Source: CAD feature listing. Evaluate the final solid. Frame: model axes, mm. A direction names the side the tool comes from. Round coordinates to 2 decimals unless told otherwise and drop trailing zeros. Write each loop counter-clockwise with the first axis right and the second up, starting at its lowest first coordinate (ties: lowest second). Pieces come first, ordered by that corner, then holes. Notation, with made-up numbers: M 62.5,70.25 L 100.5,70.25 A14 ccw 100.5,84.25 Z; hole C -18.5,5.25 d4. An arc over 180 degrees is marked long. Answer in a Markdown table with one row per item.
from build123d import *

# Parameters (mm, degrees)
BOX005_W                  = 41
BOX005_H                  = 42
BOX005_DEPTH              = 40
BOX004_W                  = 7
BOX004_H                  = 17
BOX004_DEPTH              = 10
CYLINDER003_R             = 2.5
CYLINDER003_DEPTH         = 25
CYLINDER002_R             = 2.5
CYLINDER002_DEPTH         = 4
BOX006_W                  = 45
BOX006_H                  = 3
BOX006_DEPTH              = 8
BOX007_W                  = 3
BOX007_H                  = 50
BOX007_DEPTH              = 8
BOX003_W                  = 45
BOX003_H                  = 50
BOX003_DEPTH              = 3
FUSION002_ROLL_ANGLE      = 90
FUSION002_PLACEMENT_ANGLE = 90


with BuildPart() as base_motor:
    # Box005 → Box005 (new body)
    with BuildSketch(Plane(origin=(4, 4, 0), x_dir=(1, 0, 0), z_dir=(0, 0, 1))):
        with Locations((20.5, 21)):
            Rectangle(BOX005_W, BOX005_H)
    extrude(amount=BOX005_DEPTH)


with BuildPart() as obj1:
    # Box004 → Box004 (new body)
    with BuildSketch(Plane(origin=(45, 16.5, 0), x_dir=(1, 0, 0), z_dir=(0, 0, 1))):
        with Locations((3.5, 8.5)):
            Rectangle(BOX004_W, BOX004_H)
    extrude(amount=BOX004_DEPTH)


with BuildPart() as motor:
    # Cylinder003 → Cylinder003 (new body)
    with BuildSketch(Plane(origin=(25, 25, 43), x_dir=(1, 0, 0), z_dir=(0, 0, 1))):
        Circle(CYLINDER003_R)
    extrude(amount=CYLINDER003_DEPTH)

    # Fusion003: union base motor, obj1
    add(base_motor.part)
    add(obj1.part)


with BuildPart() as obj2:
    # Cylinder002 → Cylinder002 (new body)
    with BuildSketch(Plane(origin=(10, 10, 43), x_dir=(1, 0, 0), z_dir=(0, 0, 1))):
        Circle(CYLINDER002_R)
    extrude(amount=CYLINDER002_DEPTH)


with BuildPart() as obj3:
    # Link003 base: copy of obj2
    add(obj2.part)


with BuildPart() as obj3_1:
    # Link003 placement: moved
    add(obj3.part.moved(Location((30, 30, 0))))


with BuildPart() as obj4:
    # Link004 base: copy of obj2
    add(obj2.part)


with BuildPart() as obj4_1:
    # Link004 placement: moved
    add(obj4.part.moved(Location((30, 0, 0))))


with BuildPart() as obj5:
    # Link005 base: copy of obj2
    add(obj2.part)


with BuildPart() as obj5_1:
    # Link005 placement: moved
    add(obj5.part.moved(Location((0, 30, 0))))


with BuildPart() as obj6:
    # Box006 → Box006 (new body)
    with BuildSketch(Plane.XY.offset(32)):
        with Locations((22.5, 1.5)):
            Rectangle(BOX006_W, BOX006_H)
    extrude(amount=BOX006_DEPTH)


with BuildPart() as lateral_der:
    # Link006 base: copy of obj6
    add(obj6.part)


with BuildPart() as lateral_der_1:
    # Link006 placement: moved
    add(lateral_der.part.moved(Location((0, 47, 0))))


with BuildPart() as obj7:
    # Box007 → Box007 (new body)
    with BuildSketch(Plane.XY.offset(32)):
        with Locations((1.5, 25)):
            Rectangle(BOX007_W, BOX007_H)
    extrude(amount=BOX007_DEPTH)


with BuildPart() as obj8:
    # Box003 → Box003 (new body)
    with BuildSketch(Plane.XY.offset(40)):
        with Locations((22.5, 25)):
            Rectangle(BOX003_W, BOX003_H)
    extrude(amount=BOX003_DEPTH)

    # Fusion004: union obj6, lateral der, obj7
    add(obj6.part)
    add(lateral_der_1.part)
    add(obj7.part)

    # Fusion002: union motor, obj3, obj4, obj5, obj2
    add(motor.part)
    add(obj3_1.part)
    add(obj4_1.part)
    add(obj5_1.part)
    add(obj2.part)


with BuildPart() as obj8_1:
    # Fusion002 roll: moved
    add(obj8.part.rotate(Axis((0, 0, 0), (1, 0, 0)), FUSION002_ROLL_ANGLE))


with BuildPart() as obj8_2:
    # Fusion002 placement: moved
    add(obj8_1.part.moved(Location((0, -22.5, 5))).rotate(Axis((0, -22.5, 5), (0, 0, 1)), FUSION002_PLACEMENT_ANGLE))


solid = obj8_2.part
Q1. Pull-direction query (Z, two-part tool) for faces 4 (the flat face through (5, 26, 38.5)), 5 (the cylindrical face through (45, 16, 43)), 6 (the flat face through (5, 26, 21.5)), 7 (the flat face through (47, -13, 45)); classes: pulls with the +Z half, pulls with the -Z half, needs draft (parallel to the pull), parting line crosses it, or undercut.
Solutions:
| item | result |
|---|---|
| face 4 | pulls with the +Z half |
| face 5 | undercut |
| face 6 | pulls with the -Z half |
| face 7 | needs draft |
Q2. Section B-B (z = 30). Return loops of the section in (x, y).
Solutions:
| item | result |
|---|---|
| outline | M 0,-18.5 L 40,-18.5 L 40,-19.5 L 32,-19.5 L 32,-22.5 L 43,-22.5 L 43,0 L 68,0 L 68,5 L 43,5 L 43,22.5 L 10,22.5 L 10,29.5 L 0,29.5 Z |
Q3. Access query for faces 1 (the flat face through (32, -20, 28)), 2 (the flat face through (10, 26, 30)), 3 (the cylindrical face through (44.97, -13.04, 12.56)). Directions: +Z, -Z, +X, -X, +Y, -Y. A direction counts if a zero-diameter tool reaches every point of the face in a straight line with its end or side. Return the directions, or none.
Solutions:
| item | result |
|---|---|
| face 1 | -X, -Y |
| face 2 | +Z, -Z, +X, +Y |
| face 3 | +X |
Q4. Section A-A (y = 2.5). Return loops of the section in (x, z), and give its area (3 significant figures).
Solutions:
| item | result |
|---|---|
| outline | M 0,9 L 40,9 L 40,8 L 32,8 L 32,5 L 43,5 L 43,27.5 L 68,27.5 L 68,32.5 L 43,32.5 L 43,55 L 32,55 L 32,52 L 40,52 L 40,51 L 0,51 Z |
| area | 2,000 mm2 |
Q5. Contact query for flat-ended pins moving along their axis: pin 1 Ø12 at (x, z) = (11.5, 22.5) entering from -Y; pin 2 Ø4 at (y, z) = (17.5, 44) entering from +X; pin 3 Ø2 at (y, z) = (-4, 13) entering from +X. Output: stop coordinate, or through.
Solutions:
| item | result |
|---|---|
| pin 1 | stops at y = -18.5 |
| pin 2 | stops at x = 47 |
| pin 3 | stops at x = 43 |
Q6. Material intervals for probe 1 along Z at (x, y) = (36, -12.5); probe 2 along Y at (x, z) = (37, 26); probe 3 along Y at (x, z) = (41, 22.5), sorted ascending.
Solutions:
| item | result |
|---|---|
| probe 1 | z = 5 to 8, 9 to 51, 52 to 55 |
| probe 2 | y = -22.5 to -19.5, -18.5 to 22.5 |
| probe 3 | y = -22.5 to 22.5 |
Q7. Section C-C (x = 19). Return loops of the section in (y, z).
Solutions:
| item | result |
|---|---|
| outline | M -18.5,9 L 22.5,9 L 22.5,51 L -18.5,51 Z |
Q8. Section D-D (z = 45). Return loops of the section in (x, y), and give its area (3 significant figures).
Solutions:
| item | result |
|---|---|
| outline | M 0,-18.5 L 40,-18.5 L 40,-19.5 L 32,-19.5 L 32,-22.5 L 43,-22.5 L 43,-15 L 47,-15 L 47,-10 L 43,-10 L 43,15 L 47,15 L 47,20 L 43,20 L 43,22.5 L 0,22.5 Z |
| area | 1,840 mm2 |
